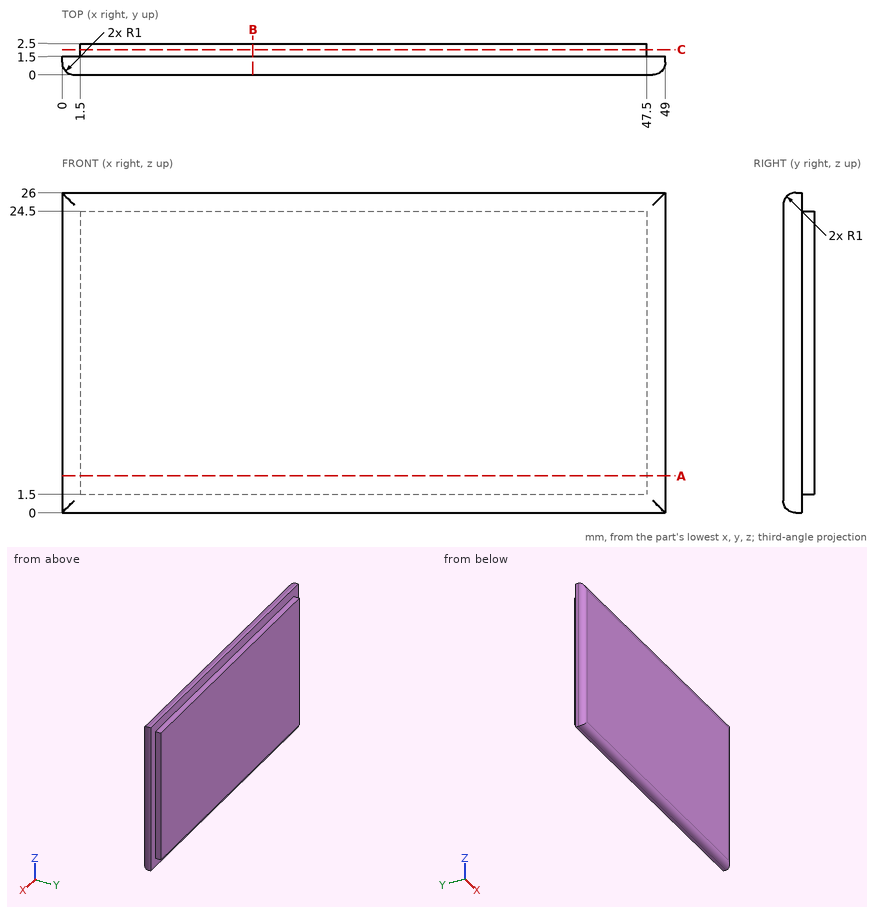
Design review of the part shown in the three views and the two pictorial views. Dimensions are in mm from the part's minimum x, y and z. Coordinates: 2 decimals unless noted, no trailing zeros. Loops run counter-clockwise (first coordinate to the right, second up) from the corner with the lowest first, then second, coordinate; pieces in that order, holes last. Notation, with made-up numbers: M 86,-27 L 125,-27 A32 cw 125,1 Z; hole C 71.25,58 d5. An arc over 180 degrees is marked long. Put each result on its own line as item: value. Start each with the question number.
Q1. Add section B-B (x = 15.5). Write out the cut boundary in (y, z), and give its area (3 significant figures).
Q2. Clearance check with flat-ended pins moving along their axes: pin 1 (0.8 mm diameter, centred on y = 2, z = 8.5, fed in from -X); pin 2 (12 mm diameter, centred on x = 27, z = 7.5, fed in from -Y); pin 3 (0.5 mm diameter, centred on x = 24, y = 2, fed in from +Z). State where each tip first meets the part, or that it passes through.
Q3. Add section A-A (z = 3). Write out the cut boundary in (x, y), and give its area (3 significant figures).
Q4. Wall thickness on line 1 (X direction, y = 0.85, z = 19.25); line 2 (X direction, y = 1.6, z = 13.75); line 3 (Z direction, x = 9.5, y = 2.2): over which ranges is each line inside the solid? List them lowest first.
Q5. Add section C-C (y = 2.05). Write out the cut boundary in (x, z).
Answers:
1. outline: M 0,1 A1 ccw 1,0 L 1.5,0 L 1.5,1.5 L 2.5,1.5 L 2.5,24.5 L 1.5,24.5 L 1.5,26 L 1,26 A1 ccw 0,25 Z
1. area: 61.6 mm^2
2. pin 1: stops at x = 1.5
2. pin 2: stops at y = 0
2. pin 3: stops at z = 24.5
3. outline: M 0,1 A1 ccw 1,0 L 48,0 A1 ccw 49,1 L 49,1.5 L 47.5,1.5 L 47.5,2.5 L 1.5,2.5 L 1.5,1.5 L 0,1.5 Z
3. area: 119 mm^2
4. line 1: x = 0.01 to 48.99
4. line 2: x = 1.5 to 47.5
4. line 3: z = 1.5 to 24.5
5. outline: M 1.5,1.5 L 47.5,1.5 L 47.5,24.5 L 1.5,24.5 Z
